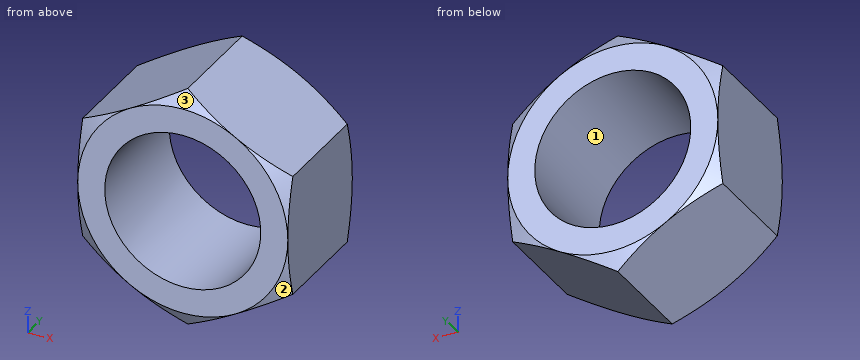
from build123d import *

# Parameters (mm, degrees)
SKETCH1_R           = 3.302
BOSS_EXTRUDE1_DEPTH = 2.54
SKETCH2_OUTSIDE_W   = 31.388
SKETCH2_OUTSIDE_H   = 32.764
SKETCH2_OUTSIDE_R   = 4.445
CUT_EXTRUDE1_DEPTH  = 5.08
CUT_EXTRUDE1_DRAFT  = -60
SKETCH3_OUTSIDE_W   = 31.388
SKETCH3_OUTSIDE_H   = 32.764
SKETCH3_OUTSIDE_R   = 4.445
CUT_EXTRUDE2_DEPTH  = 5.08
CUT_EXTRUDE2_DRAFT  = -60


with BuildPart() as part:
    # Sketch1 → Boss-Extrude1 (new, symmetric)
    with BuildSketch(Plane(origin=(0, 0, 0), x_dir=(1, 0, 0), z_dir=(0, 1, 0))):
        Polygon((0, 5.132643893), (-4.445, 2.566321947), (-4.445, -2.566321947), (0, -5.132643893), (4.445, -2.566321947), (4.445, 2.566321947), align=None)
        with Locations(Location((0, 0, 0), (0, 0, 270))):
            Circle(SKETCH1_R, mode=Mode.SUBTRACT)
    extrude(amount=BOSS_EXTRUDE1_DEPTH, both=True)


with BuildPart() as cut_extrude1_tool:
    # Sketch2 outside → Cut-Extrude1 (with draft: the straight prism first)
    with BuildSketch(Plane(origin=(0, 2.54, 0), x_dir=(1, 0, 0), z_dir=(0, 1, 0))):
        Rectangle(SKETCH2_OUTSIDE_W, SKETCH2_OUTSIDE_H)
        Circle(SKETCH2_OUTSIDE_R, mode=Mode.SUBTRACT)
    extrude(amount=-CUT_EXTRUDE1_DEPTH)
    # Cut-Extrude1: the draft: its side faces are tilted about the plane it starts from
    cut_extrude1_sides = [cut_extrude1_tool.faces().sort_by_distance(p)[0] for p in [
        (0, 0, 16.382),
        (15.694, 0, 0),
        (0, 0, -16.382),
        (-15.694, 0, 0),
        (-4.445, 0, 0),
    ]]
    draft(cut_extrude1_sides, Plane(origin=(0, 2.54, 0), x_dir=(1, 0, 0), z_dir=(0, 1, 0)), CUT_EXTRUDE1_DRAFT)


with BuildPart() as part_1:
    add(part.part)

    # Cut-Extrude1: cut by cut_extrude1_tool
    add(cut_extrude1_tool.part, mode=Mode.SUBTRACT)


with BuildPart() as cut_extrude2_tool:
    # Sketch3 outside → Cut-Extrude2 (with draft: the straight prism first)
    with BuildSketch(Plane(origin=(0, -2.54, 0), x_dir=(-1, 0, 0), z_dir=(0, -1, 0))):
        Rectangle(SKETCH3_OUTSIDE_W, SKETCH3_OUTSIDE_H)
        Circle(SKETCH3_OUTSIDE_R, mode=Mode.SUBTRACT)
    extrude(amount=-CUT_EXTRUDE2_DEPTH)
    # Cut-Extrude2: the draft: its side faces are tilted about the plane it starts from
    cut_extrude2_sides = [cut_extrude2_tool.faces().sort_by_distance(p)[0] for p in [
        (0, 0, 16.382),
        (-15.694, 0, 0),
        (0, 0, -16.382),
        (15.694, 0, 0),
        (4.445, 0, 0),
    ]]
    draft(cut_extrude2_sides, Plane(origin=(0, -2.54, 0), x_dir=(-1, 0, 0), z_dir=(0, -1, 0)), CUT_EXTRUDE2_DRAFT)


with BuildPart() as part_2:
    add(part_1.part)

    # Cut-Extrude2: cut by cut_extrude2_tool
    add(cut_extrude2_tool.part, mode=Mode.SUBTRACT)


solid = part_2.part
Build history of the part. All positions in model axes, mm. Face numbers are marked on the shaded views. Round coordinates to 2 decimals unless told otherwise and drop trailing zeros. Loops run counter-clockwise (first coordinate to the right, second up) from the corner with the lowest first, then second, coordinate; pieces in that order, holes last. Notation, with made-up numbers: (-2.5, -31) -> (20.5, -31) arc R9 ccw to (20.5, -22) -> close; hole circle Ø5 at (74, 26.25). An arc over 180 degrees is marked (long way). Use CSV: the item, a comma, the result in double quotes. Start each with the question number.
Q1. Drill centre lines: L1, parallel to X at y = -1.3, z = 0 (3 decimals); L2, parallel to X at y = -1.75, z = 1 (3 decimals); L3, parallel to Z at x = -3, y = -0.5. Where is each one in solid material? Low to high.
Q2. Saw through at A-A on y = -1.35. Give the cut face in (x, z) (3 decimals), and give its area (3 significant figures).
Q3. Mould opens along X. For the marked faces 1, 2 and 3 say: +X half, -X half, draft (parallel to the pull), parting line (faces both ways), or undercut.
Q4. Flat gauge pins, fed straight in: pin 1 Ø1 at (x, y) = (2.5, 2) entering from -Z; pin 2 Ø3 at (y, z) = (-1, -3.5) entering from -X (3 decimals); pin 3 Ø1.5 at (x, y) = (2, 1) entering from +Z. Where does each tip first touch, or does it go through?
Solutions:
1,L1,"x = -4.445 to -3.302, 3.302 to 4.445"
1,L2,"x = -4.445 to -3.147, 3.147 to 4.445"
1,L3,"z = -3.4 to -1.38, 1.38 to 3.4"
2,outline,"(-4.445, -2.566) -> (0, -5.133) -> (4.445, -2.566) -> (4.445, 2.566) -> (0, 5.133) -> (-4.445, 2.566) -> close; hole circle Ø6.604 at (0, 0)"
2,area,"34.2 mm^2"
3,face 1,"undercut"
3,face 2,"+X half"
3,face 3,"parting line"
4,pin 1,"stops at z = -3.98"
4,pin 2,"stops at x = -4.445"
4,pin 3,"stops at z = 4.41"
